from build123d import *

# Parameters (mm, degrees)
SKETCH1_R                      = 9.9375
SKETCH1_R_2                    = 6.35
SKETCH1_R_3                    = 0.5
BOSS_EXTRUDE1_DEPTH            = 6.35
F_8_0_199_DIAMETER_HOLE1_D     = 5.0546
F_8_0_199_DIAMETER_HOLE1_DEPTH = 8.35
F_8_0_199_DIAMETER_HOLE1_TIP   = 1.518555042


with BuildPart() as part:
    # Sketch1 → Boss-Extrude1 (new body)
    with BuildSketch(Plane.XY):
        Circle(SKETCH1_R)
        Circle(SKETCH1_R_2, mode=Mode.SUBTRACT)
        with Locations((-7.9375, 0)):
            Circle(SKETCH1_R_3, mode=Mode.SUBTRACT)
        with Locations((-3.96875, 6.874076643)):
            Circle(SKETCH1_R_3, mode=Mode.SUBTRACT)
        with Locations((3.96875, 6.874076643)):
            Circle(SKETCH1_R_3, mode=Mode.SUBTRACT)
        with Locations((7.9375, 0)):
            Circle(SKETCH1_R_3, mode=Mode.SUBTRACT)
        with Locations((3.96875, -6.874076643)):
            Circle(SKETCH1_R_3, mode=Mode.SUBTRACT)
        with Locations((-3.96875, -6.874076643)):
            Circle(SKETCH1_R_3, mode=Mode.SUBTRACT)
    extrude(amount=BOSS_EXTRUDE1_DEPTH)

    # #8 (0.199) Diameter Hole1
    with Locations(Plane.XZ.offset(9.9375)):
        with Locations((0, 3.175)):
            Hole(F_8_0_199_DIAMETER_HOLE1_D / 2, depth=F_8_0_199_DIAMETER_HOLE1_DEPTH)
            with Locations((0, 0, -(F_8_0_199_DIAMETER_HOLE1_DEPTH + F_8_0_199_DIAMETER_HOLE1_TIP / 2))):  # 118° drill point
                Cone(0, F_8_0_199_DIAMETER_HOLE1_D / 2, F_8_0_199_DIAMETER_HOLE1_TIP, mode=Mode.SUBTRACT)


solid = part.part
Verification items for the finished model (mm, model axes). Coordinates: 2 decimals unless noted, no trailing zeros. Order: outer loops, then holes, each group sorted by start corner. A loop starts at its lowest first (then second) coordinate and runs counter-clockwise, first axis right, second up. Notation, with made-up numbers: M 39,11 L 67,11 A28 cw 67,49 Z; hole C 67,60 d9. An arc over 180 degrees is marked long. One line per item, written item: value. Start each with the question number.
Item 1: Sectioned sample at A-A (x = 0). Enter the section's corners in (y, z).
Item 2: Sectioned sample at D-D (x = 8). Enter the section's corners in (y, z).
Item 3: Sectioned sample at C-C (z = 4.5). Count the separate pieces of the cut face and the enclosed holes in it, then the cut area to 3 significant figures.
Item 4: Mould release check, pull along Y, two halves, no side actions. Record for faces 1 (the cylindrical face through (-1.294, 9.853, 3.131)), 2 (the cylindrical face through (8.4, -0.19, 3.13)), 3 (the cylindrical face through (2.01, -7.86, 1.64)), 4 (the cylindrical face through (3.572, -7.178, 3.131)): released by +Y, released by -Y, zero draft, split by the parting line, or undercut.
Item 5: Gauge pin test, flat ends, axial feed: pin 1 (1 mm diameter, centred on x = 5.5, z = 3.5, fed in from +Y); pin 2 (3 mm diameter, centred on x = -2, z = 3.5, fed in from -Y). Record the tip position at first contact, or that the pin passes through.
Item 6: Sectioned sample at B-B (y = 0). Enter the section's corners in (x, z).
Item 7: Scan lines: probe 1 along X at (y, z) = (6.75, 6); probe 2 along Y at (x, z) = (4, 3.5); probe 3 along X at (y, z) = (2, 4). Record each from-to range of solid material in increasing order.
Conclusion:
1. outline: M -9.94,0 L -6.35,0 L -6.35,0.65 L -9.94,0.65 Z; M -9.94,5.7 L -6.35,5.7 L -6.35,6.35 L -9.94,6.35 Z; M 6.35,0 L 9.94,0 L 9.94,6.35 L 6.35,6.35 Z
2. outline: M -5.9,0 L -0.5,0 L -0.5,6.35 L -5.9,6.35 Z; M 0.5,0 L 5.9,0 L 5.9,6.35 L 0.5,6.35 Z
3. separate pieces: 1
3. enclosed holes: 6
3. area: 163 mm^2
4. face 1: split by the parting line
4. face 2: undercut
4. face 3: zero draft
4. face 4: undercut
5. pin 1: stops at y = 8.59
5. pin 2: stops at y = -9.78
6. outline: M -9.94,0 L -8.44,0 L -8.44,6.35 L -9.94,6.35 Z; M -7.44,0 L -6.35,0 L -6.35,6.35 L -7.44,6.35 Z; M 6.35,0 L 7.44,0 L 7.44,6.35 L 6.35,6.35 Z; M 8.44,0 L 9.94,0 L 9.94,6.35 L 8.44,6.35 Z
7. probe 1: x = -7.29 to -4.45, -3.48 to 3.48, 4.45 to 7.29
7. probe 2: y = -9.1 to -7.37, -6.38 to -4.93, 4.93 to 6.38, 7.37 to 9.1
7. probe 3: x = -9.73 to -6.03, 6.03 to 9.73
